```python
from build123d import *

# Parameters (mm, degrees)
F0_W     = 243.84
F0_H     = 304.8
F1_DEPTH = 3.175
F3_D     = 3.9624
F4_W     = 22.606
F4_H     = 158.75
F5_DEPTH = 44.45


with BuildPart() as f1:
    # F0 (on Top) → F1 (new body)
    with BuildSketch(Plane.XY):
        with Locations((-121.92, -152.4)):
            Rectangle(F0_W, F0_H)
    extrude(amount=F1_DEPTH)

    # F3 (through all)
    with Locations(Plane.XY.offset(3.175)):
        with Locations((-78.74, -10.16), (-210.82, -10.16), (-6.35, -10.16), (-78.74, -292.1), (-78.74, -167.64), (-6.35, -292.1), (-233.68, -167.64), (-233.68, -292.1), (-6.35, -167.64), (-233.68, -213.36)):
            Hole(F3_D / 2)

    # F4 (on face) → F5 (join)
    with BuildSketch(Plane.XY.offset(3.175)):
        with Locations((-233.68, -78.7654)):
            Rectangle(F4_W, F4_H)
    extrude(amount=F5_DEPTH)


solid = f1.part
```
The listing builds one solid part. Answer for the finished solid, in the listing's coordinates (mm). A direction names the side the tool comes from. Coordinates: 2 decimals unless noted, no trailing zeros. Loops run counter-clockwise (first coordinate to the right, second up) from the corner with the lowest first, then second, coordinate; pieces in that order, holes last. Notation, with made-up numbers: M 85.5,33 L 136.5,33 A15 cw 136.5,39 Z; hole C 23.5,34.25 d8. An arc over 180 degrees is marked long. Answer as CSV lines item,"result". Start each with the question number.
(1) For faces 1 (the flat face through (-222.377, -80, 25)), 2 (the flat face through (-234, 0.61, 25)), 3 (the flat face through (-234, -158.14, 25)), determine the directions among +Z, -Z, +X, -X, +Y, -Y from which every point of the face is accessible in a straight line to the end or side of a thin tool.
(2) The part is cut by section B-B (z = 32). Give the vertices of the cut face in (x, y), and give its area (3 significant figures).
(3) Given pin 1 (13.5 mm diameter, centred on y = -62.5, z = 36.5, fed in from +X); pin 2 (3 mm diameter, centred on x = -77, y = -183.5, fed in from +Z) (3 decimals); pin 3 (2.5 mm diameter, centred on x = -167, z = 1.5, fed in from +Y), each flat-ended and moving along its own axis, determine where each tip first touches the part or whether it passes through.
(4) The part is cut by section A-A (y = -31). Give the vertices of the cut face in (x, z) (3 decimals), and give its area (3 significant figures).
(5) The part is cut by section C-C (x = -160). Give the vertices of the cut face in (y, z) (3 decimals), and give its area (3 significant figures).
(6) Find the intervals of material crossed by L1, parallel to X at y = -167.64, z = 0.95; L2, parallel to Y at x = -210.82, z = 2.1; L3, parallel to Y at x = -227.5, z = 23, in increasing order. Write a range as [from, to].
Determined:
1,face 1,"+Z, +X, +Y, -Y"
1,face 2,"+Z, -Z, +X, -X, +Y"
1,face 3,"+Z, +X, -X, -Y"
2,outline,"M -244.98,-158.14 L -222.38,-158.14 L -222.38,0.61 L -244.98,0.61 Z"
2,area,"3,590 mm2"
3,pin 1,"x = -222.38"
3,pin 2,"z = 3.175"
3,pin 3,"y = 0"
4,outline,"M -244.983,3.175 L -243.84,3.175 L -243.84,0 L 0,0 L 0,3.175 L -222.377,3.175 L -222.377,47.625 L -244.983,47.625 Z"
4,area,"1,780 mm2"
5,outline,"M -304.8,0 L 0,0 L 0,3.175 L -304.8,3.175 Z"
5,area,"968 mm2"
6,L1,"[-243.84, -235.66], [-231.7, -80.72], [-76.76, -8.33], [-4.37, 0]"
6,L2,"[-304.8, -12.14], [-8.18, 0]"
6,L3,"[-158.14, 0.61]"
